Geometry check sheet. Reference: the model listing, model coordinates, mm. A direction names the side the tool comes from. Coordinates: 2 decimals unless noted, no trailing zeros. Write each loop counter-clockwise with the first axis right and the second up, starting at its lowest first coordinate (ties: lowest second). Pieces come first, ordered by that corner, then holes. Notation, with made-up numbers: (84, 13.25) -> (135, 13.25) arc R10 cw to (135, 27.25) -> close; hole circle Ø6 at (85, -1). An arc over 180 degrees is marked (long way). One line per question, with ' | ' between items.
from build123d import *

# Parameters (mm, degrees)
F0_R     = 12.7
F1_DEPTH = 25.4
F2_R     = 3.175
F3_DEPTH = 12.7


with BuildPart() as f1:
    # F0 (on Front) → F1 (new body)
    with BuildSketch(Plane.XZ):
        with BuildLine():
            Line((-14.600585, 25.4), (-14.600585, 0))
            Line((-14.600585, 0), (23.499415, 0))
            Line((23.499415, 0), (23.499415, 25.4))
            ThreePointArc((23.499415, 25.4), (4.449415, 44.45), (-14.600585, 25.4))
        make_face()
        with Locations((4.449415, 25.4)):
            Circle(F0_R, mode=Mode.SUBTRACT)
    extrude(amount=F1_DEPTH)

    # F2 (on face) → F3 (cut)
    with BuildSketch(Plane(origin=(0, 0, 0), x_dir=(1, 0, 0), z_dir=(0, 0, -1))):
        with Locations((-8.250585, 12.7)):
            Circle(F2_R)
        with Locations((17.149415, 12.7)):
            Circle(F2_R)
    extrude(amount=-F3_DEPTH, mode=Mode.SUBTRACT)


solid = f1.part
1. Go/stop test with flat-tipped pins: P1, Ø1, axis at x = 17, y = -12.5, coming from the -Z side; P2, Ø1, axis at x = 1, y = -20, coming from the +Z side; P3, Ø6, axis at y = -11.5, z = 32, coming from the -X side. Record where each tip stops, or that it passes through.
Worked answers:
P1: z = 12.7 | P2: z = 44.22 | P3: x = -14.26
2. Cross-section at B-B on y = -21.75. Record the boundary of the cut face in (x, z).
Worked answers:
outline: (-14.6, 0) -> (23.5, 0) -> (23.5, 25.4) arc R19.05 ccw to (-14.6, 25.4) -> close; hole circle Ø25.4 at (4.45, 25.4)
3. Cross-section at C-C on x = 12. Record the boundary of the cut face in (y, z), and give its area (3 significant figures).
Worked answers:
outline: (-25.4, 0) -> (0, 0) -> (0, 15.19) -> (-25.4, 15.19) -> close; (-25.4, 35.61) -> (0, 35.61) -> (0, 42.89) -> (-25.4, 42.89) -> close | area: 571 mm²
4. Cross-section at D-D on z = 21.5. Record the boundary of the cut face in (x, y), and give its area (3 significant figures).
Worked answers:
outline: (-14.6, -25.4) -> (-7.64, -25.4) -> (-7.64, 0) -> (-14.6, 0) -> close; (16.54, -25.4) -> (23.5, -25.4) -> (23.5, 0) -> (16.54, 0) -> close | area: 354 mm²
5. Material ranges on line 1 (X direction, y = -12.7, z = 8.5); line 2 (X direction, y = -10.25, z = 9.5); line 3 (Z direction, x = 1, y = -8.25), recorded low to high. Write a range as from..to.
Worked answers:
line 1: -14.6..-11.43, -5.08..13.97, 20.32..23.5 | line 2: -14.6..-10.27, -6.23..15.13, 19.17..23.5 | line 3: 0..13.18, 37.62..44.14
6. Cross-section at A-A on z = 10. Record the boundary of the cut face in (x, y) (3 decimals), and give its area (3 significant figures).
Worked answers:
outline: (-14.601, -25.4) -> (23.499, -25.4) -> (23.499, 0) -> (-14.601, 0) -> close; hole circle Ø6.35 at (-8.251, -12.7); hole circle Ø6.35 at (17.149, -12.7) | area: 904 mm²
7. Mould release check, pull along Y, two halves, no side actions. Record for faces 3 (the face through (0, -25.4, 13)), 4 (the face through (17, -13, 12.7)), 5 (the face through (4.868, -12.522, 44.445)): released by +Y, released by -Y, zero draft, split by the parting line, or undercut.
Worked answers:
face 3: released by -Y | face 4: undercut | face 5: zero draft
8. Tool access check on faces 1 (the face through (-8, -13, 12.7)), 2 (the face through (23.499, -13, 13)). Record the directions out of +Z, -Z, +X, -X, +Y, -Y that give a thin tool (end or side, any length) a straight path to the whole face; none if there is none.
Worked answers:
face 1: -Z | face 2: +Z, -Z, +X, +Y, -Y
